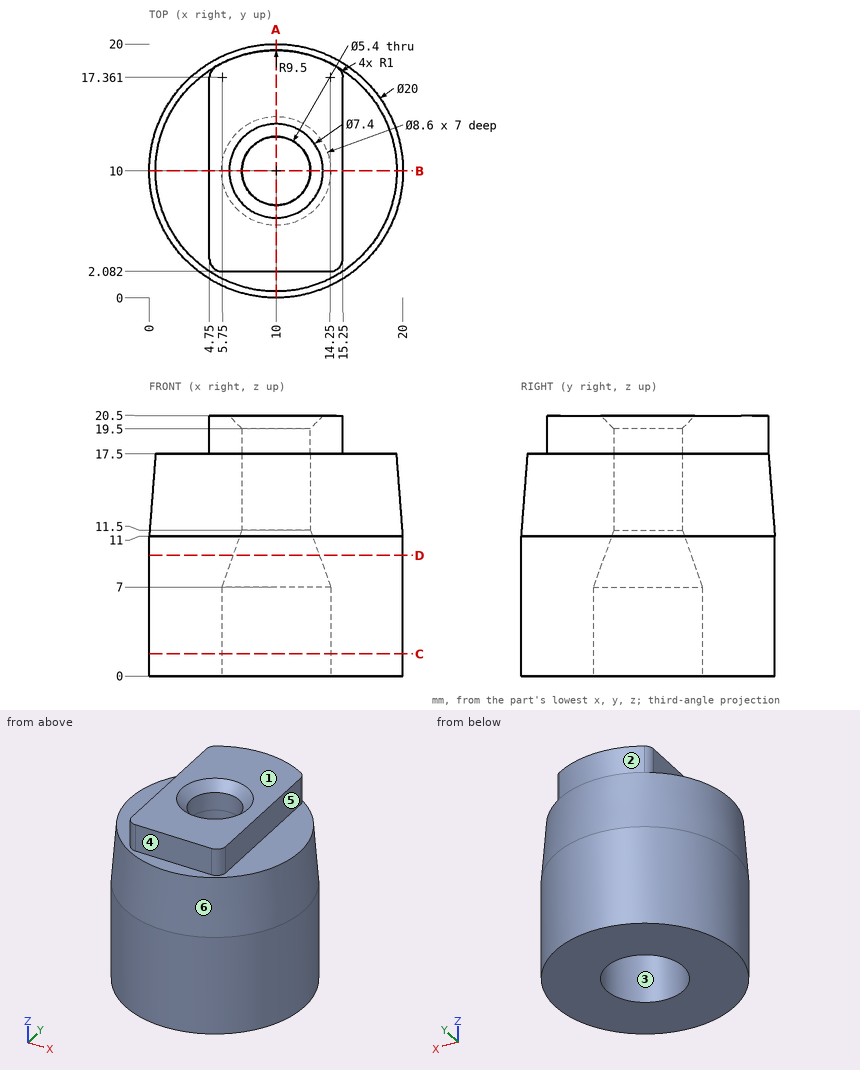
Geometry check sheet. Reference: drawing and pictorial views, mm from the part's lowest x, y, z. A direction names the side the tool comes from. Coordinates: 2 decimals unless noted, no trailing zeros. Loops run counter-clockwise (first coordinate to the right, second up) from the corner with the lowest first, then second, coordinate; pieces in that order, holes last.
1) Sectioned sample at C-C (z = 1.75). Record the boundary of the cut face in (x, y).
2) Sectioned sample at D-D (z = 9.5). Record the boundary of the cut face in (x, y).
3) Access from +Z, -Z, +X, -X, +Y, -Y to the whole of each face (thin tool, end or side, straight path). Record for the marked faces 4, 5 and 6.
4) Material ranges on probe 1 along Y at (x, z) = (10, 5.5); probe 2 along Y at (x, z) = (10, 18.65); probe 3 along X at (y, z) = (9.75, 4.5), recorded low to high.
5) Release check for a two-part mould opening along Y. For the marked faces 1, 2 and 3 record: released by +Y, released by -Y, zero draft, split by the parting line, or undercut.
6) Gauge pin test, flat ends, axial feed: pin 1 (5 mm diameter, centred on x = 16, z = 16.5, fed in from +Y) (1 decimal); pin 2 (3.5 mm diameter, centred on x = 9, z = 18.5, fed in from -Y); pin 3 (1 mm diameter, centred on x = 14.5, z = 13.5, fed in from +Y); pin 4 (5 mm diameter, centred on x = 10, y = 10, fed in from -Z). Record the tip position at first contact, or that the pin passes through.
7) Sectioned sample at B-B (y = 10). Record the boundary of the cut face in (x, z), and give its area (3 significant figures).
8) Sectioned sample at A-A (x = 10). Record the boundary of the cut face in (y, z), and give its area (3 significant figures).
Check sheet entries:
1. outline: circle Ø20 at (10, 10); hole circle Ø8.6 at (10, 10)
2. outline: circle Ø20 at (10, 10); hole circle Ø6.82 at (10, 10)
3. face 4: +Z, +X, -X, -Y
3. face 5: +Z, +X, +Y, -Y
3. face 6: +Z
4. probe 1: y = 0 to 5.7, 14.3 to 20
4. probe 2: y = 2.08 to 7.3, 12.7 to 19.5
4. probe 3: x = 0 to 5.71, 14.29 to 20
5. face 1: zero draft
5. face 2: released by +Y
5. face 3: undercut
6. pin 1: stops at y = 18.9
6. pin 2: stops at y = 0.46
6. pin 3: stops at y = 18.96
6. pin 4: passes through
7. outline: (0, 0) - (5.7, 0) - (5.7, 7) - (7.3, 11.5) - (7.3, 19.5) - (6.3, 20.5) - (4.75, 20.5) - (4.75, 17.5) - (0.5, 17.5) - (0, 11) - close; (12.7, 11.5) - (14.3, 7) - (14.3, 0) - (20, 0) - (20, 11) - (19.5, 17.5) - (15.25, 17.5) - (15.25, 20.5) - (13.7, 20.5) - (12.7, 19.5) - close
7. area: 237 mm2
8. outline: (0, 0) - (5.7, 0) - (5.7, 7) - (7.3, 11.5) - (7.3, 19.5) - (6.3, 20.5) - (2.08, 20.5) - (2.08, 17.5) - (0.5, 17.5) - (0, 11) - close; (12.7, 11.5) - (14.3, 7) - (14.3, 0) - (20, 0) - (20, 11) - (19.5, 17.5) - (19.5, 20.5) - (13.7, 20.5) - (12.7, 19.5) - close
8. area: 258 mm2
